Geometry: final body of the model. Coordinates: model frame, mm. A direction names the side the tool comes from. Coordinates: 2 decimals unless noted, no trailing zeros. Order: outer loops, then holes, each group sorted by start corner. A loop starts at its lowest first (then second) coordinate and runs counter-clockwise, first axis right, second up. Notation, with made-up numbers: M -22.75,-19.75 L 3.25,-19.75 A14 cw 3.25,5.25 Z; hole C 63.5,-14.75 d7. An arc over 180 degrees is marked long. Write item = value, one per line.
from build123d import *

# Parameters (mm, degrees)
BOSS_EXTRUDE1_DEPTH   = 25
BOSS_EXTRUDE1_2_DEPTH = 25
SKETCH1_3_W           = 176
SKETCH1_3_H           = 90
BOSS_EXTRUDE2_DEPTH   = 19
BOSS_EXTRUDE3_DEPTH   = 12
CUT_EXTRUDE1_DEPTH    = 6
CUT_EXTRUDE2_REACH    = 223.077
SKETCH2_W             = 7
SKETCH2_H             = 6
M8X1_0_TAPPED_HOLE1_D = 7
LPATTERN1_COUNT       = 2
LPATTERN1_PITCH       = 50
LPATTERN1_COUNT_DIR2  = 2
LPATTERN1_PITCH_DIR2  = 144
FILLET1_R             = 5


with BuildPart() as part:
    # Sketch1 → Boss-Extrude1 (new body)
    with BuildSketch(Plane(origin=(0, 0, 0), x_dir=(1, 0, 0), z_dir=(0, 1, 0))):
        Polygon((95, 45), (88, 45), (88, -45), (95, -45), (95, -25), (95, 25), align=None)
    extrude(amount=BOSS_EXTRUDE1_DEPTH)



with BuildPart() as body_2:
    # Sketch1 → Boss-Extrude1 2 (new body)
    with BuildSketch(Plane(origin=(0, 0, 0), x_dir=(1, 0, 0), z_dir=(0, 1, 0))):
        Polygon((-88, -45), (-88, 45), (-95, 45), (-95, 25), (-95, -25), (-95, -45), align=None)
    extrude(amount=BOSS_EXTRUDE1_2_DEPTH)


with BuildPart() as part_1:
    add(part.part)

    add(body_2.part)  # Boss-Extrude2 merges body 2
    # Sketch1<3> → Boss-Extrude2 (add)
    # profile 1 of 2: a face of its own
    with BuildSketch(Plane(origin=(0, 0, 0), x_dir=(1, 0, 0), z_dir=(0, 1, 0))):
        Rectangle(SKETCH1_3_W, SKETCH1_3_H)
        with BuildLine():
            ThreePointArc((-82, 25), (-80.535533906, 28.535533906), (-77, 30))
            Line((-77, 30), (77, 30))
            ThreePointArc((77, 30), (80.535533906, 28.535533906), (82, 25))
            Line((82, 25), (82, -25))
            ThreePointArc((82, -25), (80.535533906, -28.535533906), (77, -30))
            Line((77, -30), (-77, -30))
            ThreePointArc((-77, -30), (-80.535533906, -28.535533906), (-82, -25))
            Line((-82, -25), (-82, 25))
        make_face(mode=Mode.SUBTRACT)
    # profile 2 of 2: a face of its own
    with BuildSketch(Plane(origin=(0, 0, 0), x_dir=(1, 0, 0), z_dir=(0, 1, 0))):
        with BuildLine():
            Line((-77, 30), (77, 30))
            ThreePointArc((77, 30), (80.535533906, 28.535533906), (82, 25))
            Line((82, 25), (82, -25))
            ThreePointArc((82, -25), (80.535533906, -28.535533906), (77, -30))
            Line((77, -30), (-77, -30))
            ThreePointArc((-77, -30), (-80.535533906, -28.535533906), (-82, -25))
            Line((-82, -25), (-82, 25))
            ThreePointArc((-82, 25), (-80.535533906, 28.535533906), (-77, 30))
        make_face()
    extrude(amount=BOSS_EXTRUDE2_DEPTH)

    # Sketch1<4> → Boss-Extrude3 (add)
    with BuildSketch(Plane(origin=(0, 0, 0), x_dir=(1, 0, 0), z_dir=(0, 1, 0))):
        with BuildLine():
            Line((120, 25), (95, 25))
            Line((95, 25), (95, -25))
            Line((95, -25), (120, -25))
            Line((120, -25), (120, -7))
            Line((120, -7), (108, -7))
            ThreePointArc((108, -7), (101, 0), (108, 7))
            Line((108, 7), (120, 7))
            Line((120, 7), (120, 25))
        make_face()
        with BuildLine():
            Line((-95, -25), (-95, 25))
            Line((-95, 25), (-120, 25))
            Line((-120, 25), (-120, 7))
            Line((-120, 7), (-108, 7))
            ThreePointArc((-108, 7), (-101, 0), (-108, -7))
            Line((-108, -7), (-120, -7))
            Line((-120, -7), (-120, -25))
            Line((-120, -25), (-95, -25))
        make_face()
    extrude(amount=BOSS_EXTRUDE3_DEPTH)

    # Sketch1<5> → Cut-Extrude1 (cut)
    with BuildSketch(Plane(origin=(0, 0, 0), x_dir=(1, 0, 0), z_dir=(0, 1, 0))):
        with BuildLine():
            Line((-77, 30), (77, 30))
            ThreePointArc((77, 30), (80.535533906, 28.535533906), (82, 25))
            Line((82, 25), (82, -25))
            ThreePointArc((82, -25), (80.535533906, -28.535533906), (77, -30))
            Line((77, -30), (-77, -30))
            ThreePointArc((-77, -30), (-80.535533906, -28.535533906), (-82, -25))
            Line((-82, -25), (-82, 25))
            ThreePointArc((-82, 25), (-80.535533906, 28.535533906), (-77, 30))
        make_face()
    extrude(amount=CUT_EXTRUDE1_DEPTH, mode=Mode.SUBTRACT)

    # Sketch2 → Cut-Extrude2 (cut, up to next)
    with BuildSketch(Plane(origin=(95, 0, 0), x_dir=(0, 0, -1), z_dir=(1, 0, 0)), mode=Mode.PRIVATE) as cut_extrude2_sk1:
        with Locations((41.5, 9)):
            Rectangle(SKETCH2_W, SKETCH2_H)
    cut_extrude2_tool1 = extrude(cut_extrude2_sk1.sketch, amount=-CUT_EXTRUDE2_REACH, mode=Mode.PRIVATE) & part_1.part
    # Sketch2 → Cut-Extrude2 (cut, up to next)
    with BuildSketch(Plane(origin=(95, 0, 0), x_dir=(0, 0, -1), z_dir=(1, 0, 0)), mode=Mode.PRIVATE) as cut_extrude2_sk2:
        with Locations((-41.5, 9)):
            Rectangle(SKETCH2_W, SKETCH2_H)
    cut_extrude2_tool2 = extrude(cut_extrude2_sk2.sketch, amount=-CUT_EXTRUDE2_REACH, mode=Mode.PRIVATE) & part_1.part
    add(cut_extrude2_tool1.solids().sort_by_distance((95, 9, -41.5))[0], mode=Mode.SUBTRACT)
    add(cut_extrude2_tool2.solids().sort_by_distance((95, 9, 41.5))[0], mode=Mode.SUBTRACT)

    # M8x1.0 Tapped Hole1 (through all)
    with Locations(Plane(origin=(0, 19, 0), x_dir=(1, 0, 0), z_dir=(0, 1, 0))):
        with Locations((72, -25)):
            m8x1_0_tapped_hole1 = Hole(M8X1_0_TAPPED_HOLE1_D / 2)

    # LPattern1: M8x1.0 Tapped Hole1 2 × 2
    with Locations(*[(-j * LPATTERN1_PITCH_DIR2, 0, -i * LPATTERN1_PITCH) for i in range(LPATTERN1_COUNT) for j in range(LPATTERN1_COUNT_DIR2) if (i, j) != (0, 0)]):
        add(m8x1_0_tapped_hole1, mode=Mode.SUBTRACT)

    # Fillet1
    fillet1_edges = [part_1.edges().sort_by_distance(p)[0] for p in [
        (120, 6, -25),
        (95, 6, -25),
        (95, 6, 25),
        (120, 6, 25),
        (-120, 6, 25),
        (-95, 6, 25),
        (-95, 6, -25),
        (-120, 6, -25),
    ]]
    fillet(fillet1_edges, radius=FILLET1_R)


solid = part_1.part
1) Mould query, pull axis Z, two halves, no side actions, for faces 1 (the face through (-108, 6, 25)), 2 (the face through (88, 22, -1)), 3 (the face through (-82, 3, 0)). Classes: pulls with the +Z half, pulls with the -Z half, needs draft (parallel to the pull), parting line crosses it, or undercut.
Numbers:
face_1 = pulls with the +Z half
face_2 = needs draft
face_3 = undercut
2) Line query: L1, parallel to Z at x = -72, y = 16.5; L2, parallel to Z at x = 72, y = 10.25; L3, parallel to Z at x = 46.5, y = 3. Output: solid intervals per line, ascending.
Numbers:
L1 = -45 to -28.5, -21.5 to 21.5, 28.5 to 45
L2 = -38 to -28.5, -21.5 to 21.5, 28.5 to 38
L3 = -45 to -30, 30 to 45
3) Pin query (flat end, axial travel): pin 1 (4 mm diameter, centred on y = 20, z = 10, fed in from -X); pin 2 (13 mm diameter, centred on x = -112, y = 8.5, fed in from -Z); pin 3 (7.5 mm diameter, centred on x = 38.5, z = -41, fed in from +Y). Return the tip coordinate at first contact, or that it passes through.
Numbers:
pin_1 = -95
pin_2 = -25
pin_3 = 19
4) Section B-B, the plane y = 16.25. Return loops of the section in (x, z).
Numbers:
outline = M -95,-45 L 95,-45 L 95,45 L -95,45 Z; hole C -72,-25 d7; hole C -72,25 d7; hole C 72,-25 d7; hole C 72,25 d7
5) Section D-D, the plane z = 0. Return loops of the section in (x, y).
Numbers:
outline = M -101,0 L -82,0 L -82,6 L 82,6 L 82,0 L 101,0 L 101,12 L 95,12 L 95,25 L 88,25 L 88,19 L -88,19 L -88,25 L -95,25 L -95,12 L -101,12 Z
6) Section C-C, the plane x = -48. Return loops of the section in (y, z), and give its area (3 significant figures).
Numbers:
outline = M 0,-45 L 6,-45 L 6,-38 L 12,-38 L 12,-45 L 19,-45 L 19,45 L 12,45 L 12,38 L 6,38 L 6,45 L 0,45 L 0,30 L 6,30 L 6,-30 L 0,-30 Z
area = 1,270 mm²
7) Section A-A, the plane x = 72. Return loops of the section in (y, z).
Numbers:
outline = M 0,-45 L 6,-45 L 6,-38 L 12,-38 L 12,-45 L 19,-45 L 19,-28.5 L 6,-28.5 L 6,-30 L 0,-30 Z; M 0,30 L 6,30 L 6,28.5 L 19,28.5 L 19,45 L 12,45 L 12,38 L 6,38 L 6,45 L 0,45 Z; M 6,-21.5 L 19,-21.5 L 19,21.5 L 6,21.5 Z
8) Set-up query: faces 4 (the face through (114, 6, 7)), 5 (the face through (82, 3, 0)), 6 (the face through (105, 12, -7)), 7 (the face through (-107, 6, -25)). Return all of +Z, -Z, +X, -X, +Y, -Y with unobstructed straight access to the full face (end or side cutting, diameter ignored); none if empty.
Numbers:
face_4 = +X, +Y, -Y
face_5 = -Y
face_6 = +Z, -Z, +X, +Y
face_7 = -Z, -X, +Y, -Y
